```python
from build123d import *

# Parameters (mm, degrees)
SIDE_COMB_DEPTH           = 4
SIDE_COMB_2_DEPTH         = 4
SIDE_COMB_3_DEPTH         = 4
SIDE_COMB_4_DEPTH         = 4
SIDE_SPACER_DEPTH         = 2.6
NARROW_SUPPORT_DEPTH      = 5
SCREW_TABS_DEPTH          = 7
SKETCH5_R                 = 1.75
SCREW_HOLES_DEPTH         = 7
SKETCH7_W                 = 5
SKETCH7_H                 = 3.5
GAP_FOR_SUPPORT_BAR_DEPTH = 2
SUPPORT_BAR_SIDES_DEPTH   = 8.5
SKETCH8_W                 = 7
SKETCH8_H                 = 7.5
SUPPORT_BAR_BOTTOM_DEPTH  = 2


with BuildPart() as part:
    # Sketch1 → Side comb (new body)
    with BuildSketch(Plane(origin=(0, 0, 0), x_dir=(0, 0, -1), z_dir=(1, 0, 0))):
        Polygon((3.396035042, -0.846726635), (0, 0), (0, -4.5), (3.396035042, -5.346726635), align=None)
    extrude(amount=SIDE_COMB_DEPTH)



with BuildPart() as body_2:
    # Sketch1 → Side comb 2 (new body)
    with BuildSketch(Plane(origin=(0, 0, 0), x_dir=(0, 0, -1), z_dir=(1, 0, 0))):
        Polygon((28.623723925, -7.13669592), (5.821774358, -1.451531374), (5.821774358, -5.951531374), (28.623723925, -11.63669592), align=None)
    extrude(amount=SIDE_COMB_2_DEPTH)


with BuildPart() as body_3:
    # Sketch1 → Side comb 3 (new body)
    with BuildSketch(Plane(origin=(0, 0, 0), x_dir=(0, 0, -1), z_dir=(1, 0, 0))):
        Polygon((58.70289144, -14.636274684), (31.049463241, -7.741500659), (31.049463241, -12.241500659), (58.70289144, -19.136274684), align=None)
    extrude(amount=SIDE_COMB_3_DEPTH)


with BuildPart() as body_4:
    # Sketch1 → Side comb 4 (new body)
    with BuildSketch(Plane(origin=(0, 0, 0), x_dir=(0, 0, -1), z_dir=(1, 0, 0))):
        Polygon((89.267206817, -22.256814395), (61.128630755, -15.241079423), (61.128630755, -19.741079423), (89.267206817, -26.756814395), align=None)
    extrude(amount=SIDE_COMB_4_DEPTH)


with BuildPart() as part_1:
    add(part.part)

    add(body_2.part)  # Side spacer merges body 2

    add(body_3.part)  # Side spacer merges body 3

    add(body_4.part)  # Side spacer merges body 4
    # Sketch2 → Side spacer (add)
    with BuildSketch(Plane.ZY):
        Polygon((-89.267206817, -22.256814395), (-89.267206817, -26.756814395), (11.643548715, -1.596937253), (11.643548715, 2.903062747), align=None)
    extrude(amount=SIDE_SPACER_DEPTH)

    # Sketch3 → Narrow support (add)
    with BuildSketch(Plane.ZY.offset(2.6)):
        Polygon((-89.267206817, -24.695587136), (11.643548715, 0.464290006), (11.643548715, -1.596937253), (-89.267206817, -26.756814395), align=None)
    extrude(amount=NARROW_SUPPORT_DEPTH)

    # Sketch4 → Screw tabs (add)
    with BuildSketch(Plane.ZY.offset(7.6)):
        Polygon((-89.267206817, -24.695587136), (-80.534545281, -22.518290076), (-80.534545281, -24.579517335), (-89.267206817, -26.756814395), align=None)
        Polygon((11.643548715, 0.464290006), (11.643548715, -1.596937253), (2.910887179, -3.774234313), (2.910887179, -1.713007055), align=None)
    extrude(amount=SCREW_TABS_DEPTH)

    # Sketch5 → Screw holes (cut)
    with BuildSketch(Plane(origin=(0, -2.296040631, 0.572467225), x_dir=(1, 0, 0), z_dir=(0, 0.970295726, -0.241921896))):
        with Locations((-9.85, 88.089992525)):
            Circle(SKETCH5_R)
        with Locations((-9.85, -7.910007475)):
            Circle(SKETCH5_R)
    extrude(amount=-SCREW_HOLES_DEPTH, mode=Mode.SUBTRACT)

    # Sketch7 → Gap for support bar (cut)
    with BuildSketch(Plane(origin=(0, -4.236632084, 1.056311016), x_dir=(1, 0, 0), z_dir=(0, -0.970295726, 0.241921896))):
        with Locations((-5.1, -13.839992525)):
            Rectangle(SKETCH7_W, SKETCH7_H)
    extrude(amount=-GAP_FOR_SUPPORT_BAR_DEPTH, mode=Mode.SUBTRACT)

    # Sketch6 → Support bar sides (add)
    with BuildSketch(Plane(origin=(0, -4.236632084, 1.056311016), x_dir=(1, 0, 0), z_dir=(0, -0.970295726, 0.241921896))):
        Polygon((-2.6, -12.089992525), (-7.6, -12.089992525), (-7.6, -10.089992525), (-0.6, -10.089992525), (-0.6, -17.589992525), (-7.6, -17.589992525), (-7.6, -15.589992525), (-2.6, -15.589992525), align=None)
    extrude(amount=SUPPORT_BAR_SIDES_DEPTH)

    # Sketch8 → Support bar bottom (add)
    with BuildSketch(Plane(origin=(0, -12.484145757, 3.112647129), x_dir=(1, 0, 0), z_dir=(0, -0.970295726, 0.241921896))):
        with Locations((-4.1, -13.839992525)):
            Rectangle(SKETCH8_W, SKETCH8_H)
    extrude(amount=SUPPORT_BAR_BOTTOM_DEPTH)


solid = part_1.part
```
Verification items for the finished model (mm, model axes). A direction names the side the tool comes from. Coordinates: 2 decimals unless noted, no trailing zeros. Write each loop counter-clockwise with the first axis right and the second up, starting at its lowest first coordinate (ties: lowest second). Pieces come first, ordered by that corner, then holes. Notation, with made-up numbers: (-29, -4.75) - (2, -4.75) arc R11 cw to (2, 10.25) - close; hole circle Ø4 at (-29.75, -29). An arc over 180 degrees is marked (long way). Write item = value, one per line.
Q1. Access from +Z, -Z, +X, -X, +Y, -Y to the whole of each face (thin tool, end or side, straight path). Record for faces 1 (the face through (2, -2, 0)), 2 (the face through (0, -17, -60)), 3 (the face through (-4.15, -13.51, -14.76)), 4 (the face through (-11, -3, 2.911)), 5 (the face through (-5.135, -15.826, -10.292)).
Answer:
face_1 = +Z, +X, +Y, -Y
face_2 = +X, +Y, -Y
face_3 = +X, -X, -Y
face_4 = -Z, -X, +Y, -Y
face_5 = -X
Q2. Cross-section at C-C (z = -74). Enter the section's corners in (x, y), plus the area to 3 significant figures.
Answer:
outline = (-7.6, -22.95) - (4, -22.95) - (4, -18.45) - (-2.6, -18.45) - (-2.6, -20.89) - (-7.6, -20.89) - close
area = 40.0 mm²
Q3. Material ranges on L1, parallel to X at y = -8.25, z = -30.5; L2, parallel to X at y = -18, z = -72; L3, parallel to Y at x = 0.5, z = -33, recorded low to high. Write a range as from..to.
Answer:
L1 = -2.6..0
L2 = -2.6..4
L3 = -12.73..-8.23
Q4. Cross-section at D-D (x = -4.25). Enter the section's corners in (y, z), plus the area to 3 significant figures.
Answer:
outline = (-26.76, -89.27) - (-24.7, -89.27) - (-6.07, -14.55) - (-16.26, -12.01) - (-15.41, -8.62) - (-5.22, -11.16) - (0.46, 11.64) - (-1.6, 11.64) - (-6.68, -8.73) - (-16.87, -6.19) - (-18.68, -13.47) - (-8.49, -16.01) - close
area = 250 mm²
Q5. Go/stop test with flat-tipped pins: pin 1 Ø11.5 at (y, z) = (-16, -36.5) entering from -X; pin 2 Ø1.2 at (x, y) = (2, -1.5) entering from +Z; pin 3 Ø0.7 at (y, z) = (-2, -4.5) entering from +X; pin 4 Ø2.5 at (y, z) = (-18.5, -59.5) entering from +X. Record where each tip stops, or that it passes through.
Answer:
pin_1 = -7.6
pin_2 = 0
pin_3 = 0
pin_4 = 4
Q6. Cross-section at B-B (x = -9.75). Enter the section's corners in (y, z).
Answer:
outline = (-26.76, -89.27) - (-24.7, -89.27) - (-24.03, -86.6) - (-25.97, -86.11) - close; (-25.12, -82.72) - (-23.18, -83.21) - (-22.52, -80.53) - (-24.58, -80.53) - close; (-3.77, 2.91) - (-1.71, 2.91) - (-0.81, 6.55) - (-2.75, 7.04) - close; (-1.9, 10.43) - (0.04, 9.94) - (0.46, 11.64) - (-1.6, 11.64) - close
Q7. Mould release check, pull along X, two halves, no side actions. Record for faces 6 (the face through (-11.14, -24.85, -85.81)), 7 (the face through (-11, -24, -80.535)), 8 (the face through (-0.6, -13, -11)): released by +X, released by -X, zero draft, split by the parting line, or undercut.
Answer:
face_6 = undercut
face_7 = zero draft
face_8 = released by +X
Q8. Cross-section at A-A (y = -10.25). Enter the section's corners in (x, z).
Answer:
outline = (-7.6, -31.33) - (-2.6, -31.33) - (-2.6, -41.11) - (4, -41.11) - (4, -31.05) - (0, -31.05) - (0, -28.62) - (4, -28.62) - (4, -23.06) - (-7.6, -23.06) - close; (-7.6, -15.57) - (-0.6, -15.57) - (-0.6, -7.84) - (-7.6, -7.84) - (-7.6, -9.9) - (-2.6, -9.9) - (-2.6, -13.51) - (-7.6, -13.51) - close
